Here's how the part is built. I have some questions about the finished solid (model axes, mm). A direction names the side the tool comes from. Coordinates: 2 decimals unless noted, no trailing zeros. Order: outer loops, then holes, each group sorted by start corner. A loop starts at its lowest first (then second) coordinate and runs counter-clockwise, first axis right, second up. Notation, with made-up numbers: (1.25, -34.75) - (32.25, -34.75) arc R13 cw to (32.25, -17.75) - close; hole circle Ø9 at (13.25, -27.75). An arc over 180 degrees is marked (long way). Answer as CSV lines item,"result". Start each with the question number.
Q1. For faces 1 (the face through (-12.5, -0.1, 4.3)), 2 (the face through (-1.08, -4.88, 81.47)), which set-ups out of +Z, -Z, +X, -X, +Y, -Y let a thin tool reach every point of the face, with its end or its side?
Q2. Suppose I cut it at C-C (x = 0). Please give me the cut outline in (y, z).
Q3. Suppose I cut it at D-D (x = 10.25). Please give me the cut outline in (y, z), then the cut area to 3 significant figures.
Q4. For pin 1 Ø3 at (x, z) = (-0.5, 53.5) entering from +Y; pin 2 Ø10 at (x, y) = (0, 1.5) entering from -Z; pin 3 Ø1.5 at (x, z) = (2.5, 57.5) entering from -Y; pin 4 Ø1 at (y, z) = (3, 149.5) entering from +X, each with a flat end and sliding along its axis, tell me the tip position at first contact or that it passes through.
Q5. Suppose I cut it at A-A (z = 0). Please give me the cut outline in (x, y).
Q6. Suppose I cut it at B-B (y = 0). Please give me the cut outline in (x, z), then the cut area to 3 significant figures.
Q7. Thinking about a two-plate mould opening in Z: for faces 3 (the face through (12.5, -4.3, 165.1)), 4 (the face through (-0.175, 3.905, -0.867)), which applies, released by +Z, released by -Z, zero draft, split by the parting line, or undercut?
Q8. I need wall thicknesses on line 1 (Y direction, x = -1.25, z = 165); line 2 (Z direction, x = -2.5, y = -3); line 3 (Z direction, x = 10, y = -2.5). Which ranges of each line are inside material? Lowest first, please.
from build123d import *

# Parameters (mm, degrees)
SKETCH1_R                = 5
BOSS_EXTRUDE1_DEPTH      = 165
BOSS_EXTRUDE2_DEPTH      = 12.5
BOSS_EXTRUDE2_DEPTH_BACK = 12.5
SKETCH2_R                = 10
SKETCH2_R_2              = 4
CUT_EXTRUDE1_DEPTH       = 176.73061782
CUT_EXTRUDE1_DEPTH_BACK  = 176.73061782
SKETCH2_2_R              = 4


with BuildPart() as part:
    # Sketch1 → Boss-Extrude1 (new body)
    with BuildSketch(Plane.XY):
        Circle(SKETCH1_R)
    extrude(amount=BOSS_EXTRUDE1_DEPTH)

    # Sketch2 → Boss-Extrude2 (add, two sides: drawn at the far end of the back side and taken through both)
    # profile 1 of 2: a face of its own
    with BuildSketch(Plane(origin=(0, 0, 0), x_dir=(0, 0, -1), z_dir=(1, 0, 0)).offset(-BOSS_EXTRUDE2_DEPTH_BACK)):
        with Locations((-165, 0)):
            Circle(SKETCH2_R)
        with Locations((-165, 0)):
            Circle(SKETCH2_R_2, mode=Mode.SUBTRACT)
    # profile 2 of 2: a face of its own
    with BuildSketch(Plane(origin=(0, 0, 0), x_dir=(0, 0, -1), z_dir=(1, 0, 0)).offset(-BOSS_EXTRUDE2_DEPTH_BACK)):
        with Locations(Location((0, 0, 0), (0, 0, 180))):
            Circle(SKETCH2_R)
        with Locations(Location((0, 0, 0), (0, 0, 180))):
            Circle(SKETCH2_R_2, mode=Mode.SUBTRACT)
    extrude(amount=BOSS_EXTRUDE2_DEPTH + BOSS_EXTRUDE2_DEPTH_BACK)

    # Sketch2_2 → Cut-Extrude1 (cut, two sides: drawn at the far end of the back side and taken through both)
    with BuildSketch(Plane(origin=(0, 0, 0), x_dir=(0, 0, -1), z_dir=(1, 0, 0)).offset(-CUT_EXTRUDE1_DEPTH_BACK)):
        with Locations((-165, 0)):
            Circle(SKETCH2_2_R)
        with Locations(Location((0, 0, 0), (0, 0, 180))):
            Circle(SKETCH2_2_R)
    extrude(amount=CUT_EXTRUDE1_DEPTH + CUT_EXTRUDE1_DEPTH_BACK, mode=Mode.SUBTRACT)


solid = part.part
Here are the results:
1,face 1,"+Z, -Z, -X, +Y, -Y"
1,face 2,"none"
2,outline,"(-5, 8.66) arc R10 ccw (long way) to (5, 8.66) - (5, 156.34) arc R10 ccw (long way) to (-5, 156.34) - close; hole circle Ø8 at (0, 0); hole circle Ø8 at (0, 165)"
3,outline,"circle Ø20 at (0, 0); circle Ø20 at (0, 165); hole circle Ø8 at (0, 0); hole circle Ø8 at (0, 165)"
3,area,"528 mm²"
4,pin 1,"stops at y = 5"
4,pin 2,"stops at z = -10"
4,pin 3,"stops at y = -4.68"
4,pin 4,"stops at x = 4.33"
5,outline,"(-12.5, -10) - (12.5, -10) - (12.5, -4) - (-12.5, -4) - close; (-12.5, 4) - (12.5, 4) - (12.5, 10) - (-12.5, 10) - close"
6,outline,"(-12.5, -10) - (12.5, -10) - (12.5, -4) - (-12.5, -4) - close; (-12.5, 4) - (12.5, 4) - (12.5, 10) - (5, 10) - (5, 155) - (12.5, 155) - (12.5, 161) - (-12.5, 161) - (-12.5, 155) - (-5, 155) - (-5, 10) - (-12.5, 10) - close; (-12.5, 169) - (12.5, 169) - (12.5, 175) - (-12.5, 175) - close"
6,area,"2,050 mm²"
7,face 3,"zero draft"
7,face 4,"undercut"
8,line 1,"y = -10 to -4, 4 to 10"
8,line 2,"z = -9.54 to -2.65, 2.65 to 162.35, 167.65 to 174.54"
8,line 3,"z = -9.68 to -3.12, 3.12 to 9.68, 155.32 to 161.88, 168.12 to 174.68"
